Source: CAD feature listing. Evaluate the final solid. Frame: model axes, mm. Give positions to 0.01 mm unless a question says otherwise; leave off trailing zeros. Loops run counter-clockwise (first coordinate to the right, second up) from the corner with the lowest first, then second, coordinate; pieces in that order, holes last. Notation, with made-up numbers: M 12.25,88.25 L 63.25,88.25 A22 cw 63.25,116.25 Z; hole C 54.25,20 d4. An arc over 180 degrees is marked long. Put each result on its own line as item: value.
from build123d import *

# Parameters (mm, degrees)
SKETCH1_W                  = 70
SKETCH1_H                  = 204
BOSS_EXTRUDE1_DEPTH        = 3
SKETCH2_W                  = 12
SKETCH2_H                  = 3
SKETCH2_W_2                = 10
BOSS_EXTRUDE2_DEPTH        = 3
ESQUISSE4_W                = 3
ESQUISSE4_H                = 10
ENL_V_MAT_EXTRU_3_DEPTH    = 4
R_P_TITION_LIN_AIRE2_COUNT = 10
R_P_TITION_LIN_AIRE2_PITCH = 20
ESQUISSE5_W                = 3
ESQUISSE5_H                = 3
ENL_V_MAT_EXTRU_4_DEPTH    = 3
ESQUISSE6_W                = 10
ESQUISSE6_H                = 3
BOSS_EXTRU_1_DEPTH         = 3
ESQUISSE7_W                = 10
ESQUISSE7_H                = 3
BOSS_EXTRU_2_DEPTH         = 3


with BuildPart() as part:
    # Sketch1 → Boss-Extrude1 (new body)
    with BuildSketch(Plane(origin=(0, 0, 0), x_dir=(1, 0, 0), z_dir=(0, 1, 0))):
        with Locations((35, 102)):
            Rectangle(SKETCH1_W, SKETCH1_H)
    extrude(amount=BOSS_EXTRUDE1_DEPTH)

    # Sketch2 → Boss-Extrude2 (add)
    with BuildSketch(Plane(origin=(70, 0, 0), x_dir=(0, 0, -1), z_dir=(1, 0, 0))):
        with Locations((198, 1.5)):
            Rectangle(SKETCH2_W, SKETCH2_H)
        with Locations((177, 1.5)):
            Rectangle(SKETCH2_W_2, SKETCH2_H)
        with Locations((157, 1.5)):
            Rectangle(SKETCH2_W_2, SKETCH2_H)
        with Locations((137, 1.5)):
            Rectangle(SKETCH2_W_2, SKETCH2_H)
        with Locations((117, 1.5)):
            Rectangle(SKETCH2_W_2, SKETCH2_H)
        with Locations((97, 1.5)):
            Rectangle(SKETCH2_W_2, SKETCH2_H)
        with Locations((77, 1.5)):
            Rectangle(SKETCH2_W_2, SKETCH2_H)
        with Locations((57, 1.5)):
            Rectangle(SKETCH2_W_2, SKETCH2_H)
        with Locations((37, 1.5)):
            Rectangle(SKETCH2_W_2, SKETCH2_H)
        with Locations((17, 1.5)):
            Rectangle(SKETCH2_W_2, SKETCH2_H)
    extrude(amount=BOSS_EXTRUDE2_DEPTH)

    # Esquisse4 → Enlèv. mat.-Extru.3 (cut, through all)
    with BuildSketch(Plane(origin=(0, 3, 0), x_dir=(1, 0, 0), z_dir=(0, 1, 0))):
        with Locations((36.5, 187)):
            Rectangle(ESQUISSE4_W, ESQUISSE4_H)
    enl_v_mat_extru_3 = extrude(amount=-ENL_V_MAT_EXTRU_3_DEPTH, mode=Mode.SUBTRACT)

    # Répétition linéaire2: Enlèv. mat.-Extru.3 ×10
    with Locations(*[(0, 0, i * R_P_TITION_LIN_AIRE2_PITCH) for i in range(1, R_P_TITION_LIN_AIRE2_COUNT)]):
        add(enl_v_mat_extru_3, mode=Mode.SUBTRACT)

    # Esquisse5 → Enlèv. mat.-Extru.4 (cut, through all)
    with BuildSketch(Plane(origin=(0, 0, -2), x_dir=(-1, 0, 0), z_dir=(0, 0, -1))):
        with Locations((-36.5, 1.5)):
            Rectangle(ESQUISSE5_W, ESQUISSE5_H)
    extrude(amount=-ENL_V_MAT_EXTRU_4_DEPTH, mode=Mode.SUBTRACT)

    # Esquisse6 → Boss.-Extru.1 (add)
    with BuildSketch(Plane.XY):
        with Locations((15, 1.5)):
            Rectangle(ESQUISSE6_W, ESQUISSE6_H)
        with Locations((35, 1.5)):
            Rectangle(ESQUISSE6_W, ESQUISSE6_H)
    extrude(amount=BOSS_EXTRU_1_DEPTH)

    # Esquisse7 → Boss.-Extru.2 (add)
    with BuildSketch(Plane(origin=(0, 0, -204), x_dir=(-1, 0, 0), z_dir=(0, 0, -1))):
        with Locations((-38, 1.5)):
            Rectangle(ESQUISSE7_W, ESQUISSE7_H)
        with Locations((-18, 1.5)):
            Rectangle(ESQUISSE7_W, ESQUISSE7_H)
    extrude(amount=BOSS_EXTRU_2_DEPTH)


solid = part.part
1. Material intervals for line 1 (X direction, y = 1.2, z = -91.5); line 2 (Z direction, x = 66, y = 0.25); line 3 (Z direction, x = 10.5, y = 1.9), sorted ascending. Write a range as from..to.
Found:
line 1: 0..35, 38..70
line 2: -204..0
line 3: -204..3
2. Section query B-B (y = 0.7). State how many separate pieces and enclosed holes the cut face has, plus the area to 3 significant figures.
Found:
separate pieces: 1
enclosed holes: 10
area: 14,400 mm^2
3. Section query A-A (x = 56.5). Output: boundary loops of the cut face in (y, z).
Found:
outline: M 0,-204 L 3,-204 L 3,0 L 0,0 Z
4. Contact query for flat-ended pins moving along their axis: P1, Ø1.5, axis at y = 2, z = -69, coming from the +X side; P2, Ø0.9, axis at y = 1.5, z = -29.5, coming from the -X side; P3, Ø1.5, axis at x = 59.5, y = 2, coming from the -Z side; P4, Ø1, axis at x = 56.5, y = 2, coming from the +Z side. Output: stop coordinate, or through.
Found:
P1: x = 70
P2: x = 0
P3: z = -204
P4: z = 0
